```python
from build123d import *

# Parameters (mm, degrees)
SKETCH1_R           = 4.25
BOSS_EXTRUDE1_DEPTH = 6
CUT_EXTRUDE1_DEPTH  = 4
SKETCH3_R           = 3
BOSS_EXTRUDE2_DEPTH = 15
FILLET1_R           = 0.1
FILLET2_R           = 3


with BuildPart() as part:
    # Sketch1 → Boss-Extrude1 (new body)
    with BuildSketch(Plane.XY):
        Circle(SKETCH1_R)
    extrude(amount=BOSS_EXTRUDE1_DEPTH)

    # Sketch2 → Cut-Extrude1 (cut)
    with BuildSketch(Plane.XY.offset(6)):
        Polygon((0, 2.886751346), (-2.5, 1.443375673), (-2.5, -1.443375673), (0, -2.886751346), (2.5, -1.443375673), (2.5, 1.443375673), align=None)
    extrude(amount=-CUT_EXTRUDE1_DEPTH, mode=Mode.SUBTRACT)

    # Sketch3 → Boss-Extrude2 (add)
    with BuildSketch(Plane(origin=(0, 0, 0), x_dir=(-1, 0, 0), z_dir=(0, 0, -1))):
        Circle(SKETCH3_R)
    extrude(amount=BOSS_EXTRUDE2_DEPTH)

    # Fillet1
    fillet1_edges = [part.edges().sort_by_distance(p)[0] for p in [
        (1.25, 2.165063509, 6),
        (-1.25, 2.165063509, 6),
        (-2.5, 0, 6),
        (-1.25, -2.165063509, 6),
        (1.25, -2.165063509, 6),
        (2.5, 0, 6),
        (-4.25, 0, 0),
        (-4.25, 0, 6),
    ]]
    fillet(fillet1_edges, radius=FILLET1_R)

    # Fillet2
    fillet2_edges = [part.edges().sort_by_distance(p)[0] for p in [
        (3, 0, -15),
    ]]
    fillet(fillet2_edges, radius=FILLET2_R)


solid = part.part
```
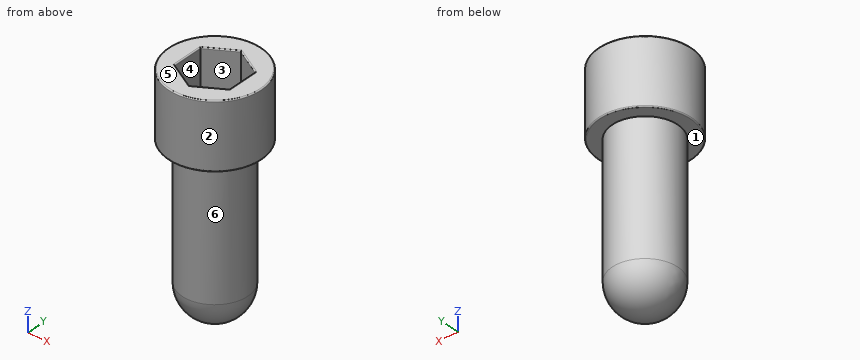
Here's how the part is built. I have some questions about the finished solid (model axes, mm). Face numbers are marked on the shaded views. A direction names the side the tool comes from. Give positions to 0.01 mm unless a question says otherwise; leave off trailing zeros. Write each loop counter-clockwise with the first axis right and the second up, starting at its lowest first coordinate (ties: lowest second). Pieces come first, ordered by that corner, then holes. Notation, with made-up numbers: M -40,35 L -17,35 A31 cw -17,60 Z; hole C 20,-33.75 d5. An arc over 180 degrees is marked long. Put each result on its own line as item: value. Start each with the question number.
Item 1: If we section it at B-B, the plane y = 0: Write out the boundary of the cut face in (x, z), then the cut area to 3 significant figures.
Item 2: Thinking about a two-plate mould opening in Y: for the marked faces 4, 5 and 6, which applies, +Y half, -Y half, draft (parallel to the pull), parting line (faces both ways), or undercut?
Item 3: On a 3-axis mill with a long thin cutter (end or side, diameter ignored), from which of +Z, -Z, +X, -X, +Y, -Y can I reach the whole of each face in a straight line? I mean the marked faces 1, 2 and 3. Say none if no direction works.
Item 4: If we section it at A-A, the plane z = 3: Write out the boundary of the cut face in (x, y).
Item 5: I need wall thicknesses on L1, parallel to Y at x = 0, z = -9.75; L2, parallel to Z at x = 0.75, y = 3; L3, parallel to X at y = -0.5, z = 4.5. Which ranges of each line are inside material? Lowest first, please. Write a range as from..to.
Item 6: If we section it at C-C, the plane z = -11.25: Write out the boundary of the cut face in (x, y), then the cut area to 3 significant figures.
Item 7: Will these pins go through, and if not, where does the flat tip stop? pin 1 (3 mm diameter, centred on y = 2.5, z = -8.5, fed in from +X); pin 2 (5 mm diameter, centred on y = 0.5, z = -4, fed in from +X); pin 3 (2.5 mm diameter, centred on x = -1, y = -0.5, fed in from -Z); pin 4 (3 mm diameter, centred on x = -3, z = 2, fed in from -Y).
Values:
1. outline: M -4.25,0.1 A0.1 ccw -4.15,0 L -3,0 L -3,-12 A3 ccw 3,-12 L 3,0 L 4.15,0 A0.1 ccw 4.25,0.1 L 4.25,5.9 A0.1 ccw 4.15,6 L 2.6,6 A0.1 ccw 2.5,5.9 L 2.5,2 L -2.5,2 L -2.5,5.9 A0.1 ccw -2.6,6 L -4.15,6 A0.1 ccw -4.25,5.9 Z
1. area: 117 mm²
2. face 4: undercut
2. face 5: draft
2. face 6: parting line
3. face 1: -Z
3. face 2: +Z, -Z
3. face 3: +Z
4. outline: C 0,0 d8.5; hole M -2.5,-1.44 L 0,-2.89 L 2.5,-1.44 L 2.5,1.44 L 0,2.89 L -2.5,1.44 Z
5. L1: -3..3
5. L2: 0..6
5. L3: -4.22..-2.5, 2.5..4.22
6. outline: C 0,0 d6
6. area: 28.3 mm²
7. pin 1: x = 2.83
7. pin 2: x = 3
7. pin 3: z = -15
7. pin 4: y = -3.98
